```python
from build123d import *

# Parameters (mm, degrees)
SKETCH1_W           = 38.1
SKETCH1_H           = 20.32
BOSS_EXTRUDE1_DEPTH = 8.89
CUT_EXTRUDE3_START  = -20.32
CUT_EXTRUDE3_DEPTH  = 20.32
CUT_EXTRUDE5_DEPTH  = 42.856889745
SKETCH15_R          = 6.9596
CUT_EXTRUDE7_DEPTH  = 31.005753887
CUT_EXTRUDE8_DEPTH  = 3.81


# Read off the part's stored shape, not the designer's step: Cut-Extrude3
with BuildPart() as part:
    # Sketch1 → Boss-Extrude1 (new body)
    with BuildSketch(Plane.XY):
        Rectangle(SKETCH1_W, SKETCH1_H)
    extrude(amount=BOSS_EXTRUDE1_DEPTH)

    # Cut-Extrude3 outline → Cut-Extrude3 (cut)
    with BuildSketch(Plane(origin=(0, 10.16, 0), x_dir=(1, 0, 0), z_dir=(0, 1, 0)).offset(CUT_EXTRUDE3_START)):
        with BuildLine():
            ThreePointArc((19.05, -6.110642457), (9.62584189, -8.191501824), (0, -8.89))
            Line((0, -8.89), (19.05, -8.89))
            Line((19.05, -8.89), (19.05, -6.110642457))
        make_face()
        with BuildLine():
            ThreePointArc((0, -8.89), (-9.62584189, -8.191501824), (-19.05, -6.110642457))
            Line((-19.05, -6.110642457), (-19.05, -8.89))
            Line((-19.05, -8.89), (0, -8.89))
        make_face()
    extrude(amount=CUT_EXTRUDE3_DEPTH, mode=Mode.SUBTRACT)

    # Sketch12 → #6 Clearance Hole2 (revolve, cut)
    with BuildSketch(Plane(origin=(13.00764722, 0, 7.608858571), x_dir=(0.9807852804032313, 0, -0.19509032201612442), z_dir=(0, 1, 0))):
        Polygon((0, 0), (0, 13.840824014), (1.89865, 12.7), (1.89865, 0), align=None)
    f_6_clearance_hole2 = revolve(axis=Axis((14.246470765, 0, 13.836845101), (-0.19509032201612442, 0, -0.9807852804032313)), mode=Mode.SUBTRACT)

    # Sketch14 → Cut-Extrude5 (cut, through all)
    with BuildSketch(Plane(origin=(12.313906035, -17.145, 4.121186114), x_dir=(-0.9807852804032313, 0, 0.19509032201612445), z_dir=(-0.19509032201612445, 0, -0.9807852804032313))):
        Polygon((0, 21.764379504), (-4.0005, 19.454689752), (-4.0005, 14.835310248), (0, 12.525620496), (4.0005, 14.835310248), (4.0005, 19.454689752), align=None)
    cut_extrude5 = extrude(amount=CUT_EXTRUDE5_DEPTH, mode=Mode.SUBTRACT)

    # Mirror1: #6 Clearance Hole2, Cut-Extrude5 across plane
    add(f_6_clearance_hole2.mirror(Plane(origin=(0, 0, 0), x_dir=(0, 0, 1), z_dir=(1, 0, 0))), mode=Mode.SUBTRACT)
    add(cut_extrude5.mirror(Plane(origin=(0, 0, 0), x_dir=(0, 0, 1), z_dir=(1, 0, 0))), mode=Mode.SUBTRACT)

    # Sketch15 → Cut-Extrude7 (cut, through all)
    with BuildSketch(Plane(origin=(-1.163639199, -10.16, 8.879845075), x_dir=(-0.9998476951563913, 0, -0.017452406437284837), z_dir=(0.017452406437284837, 0, -0.9998476951563913))):
        with Locations(Location((0, 10.16, 0), (0, 0, 180))):
            Circle(SKETCH15_R)
    extrude(amount=CUT_EXTRUDE7_DEPTH, mode=Mode.SUBTRACT)

    # Sketch16 → Cut-Extrude8 (cut)
    with BuildSketch(Plane(origin=(-1.163639199, -10.16, 8.879845075), x_dir=(-0.9998476951563913, 0, -0.017452406437284837), z_dir=(0.017452406437284837, 0, -0.9998476951563913))):
        Polygon((-4.934670486, 18.7071), (-9.869340972, 10.16), (-4.934670486, 1.6129), (4.934670486, 1.6129), (9.869340972, 10.16), (4.934670486, 18.7071), align=None)
    extrude(amount=CUT_EXTRUDE8_DEPTH, mode=Mode.SUBTRACT)


solid = part.part
```
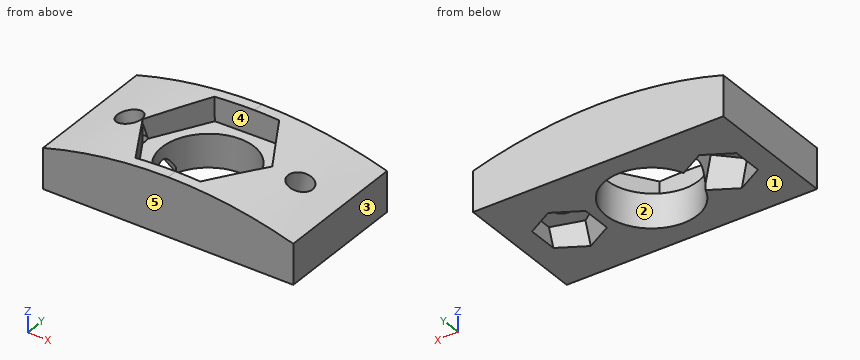
Build history of the part. All positions in model axes, mm. Face numbers are marked on the shaded views. A direction names the side the tool comes from. Round coordinates to 2 decimals unless told otherwise and drop trailing zeros. Order: outer loops, then holes, each group sorted by start corner. A loop starts at its lowest first (then second) coordinate and runs counter-clockwise, first axis right, second up. Notation, with made-up numbers: (20, 58.25) - (77, 58.25) arc R20 cw to (77, 73.25) - close; hole circle Ø1 at (14, 46.5). An arc over 180 degrees is marked (long way). Use a Markdown table: item, result.
1) Flat gauge pins, fed straight in: pin 1 Ø1.5 at (x, y) = (14.5, -2) entering from +Z; pin 2 Ø12 at (x, y) = (-14.5, 6.5) entering from -Z; pin 3 Ø5 at (x, y) = (-4.5, 2) entering from +Z. Where does each tip first touch, or does it go through?
Recorded:
| item | result |
|---|---|
| pin 1 | stops at z = 7.46 |
| pin 2 | stops at z = 0 |
| pin 3 | passes through |
2) Pull direction Y, two halves, no side cores. Call the marked faces 3, 4 and 5: pulls with the +Y half, pulls with the -Y half, needs draft (parallel to the pull), parting line crosses it, or undercut.
Recorded:
| item | result |
|---|---|
| face 3 | needs draft |
| face 4 | undercut |
| face 5 | pulls with the -Y half |
3) Wall check: L1, parallel to X at y = 4.5, z = 2; L2, parallel to X at y = -2.5, z = 2.25; L3, parallel to Y at x = 0.5, z = 8.5. Give the ranges that are in metal, low to high.
Recorded:
| item | result |
|---|---|
| L1 | x = -19.05 to -12.1, -11.68 to -6.35, 4.27 to 11.68, 12.1 to 19.05 |
| L2 | x = -19.05 to -15.68, -8.2 to -7.54, 5.45 to 8.2, 15.68 to 19.05 |
| L3 | y = -10.16 to -8.55, 8.55 to 10.16 |
4) Saw through at C-C on x = 8. Write the cut outline in (y, z), and give its area (3 significant figures).
Recorded:
| item | result |
|---|---|
| outline | (-10.16, 0) - (-2.64, 0) - (-2.31, 2.94) - (2.31, 2.94) - (2.64, 0) - (10.16, 0) - (10.16, 8.41) - (1.24, 8.41) - (1.34, 5.23) - (-1.34, 5.23) - (-1.24, 8.41) - (-10.16, 8.41) - close |
| area | 148 mm² |
5) Tool access for the marked faces 1 and 2: list every direction of +Z, -Z, +X, -X, +Y, -Y with a clear straight run to the whole face (end or side of a thin tool).
Recorded:
| item | result |
|---|---|
| face 1 | -Z, +X, -X, +Y, -Y |
| face 2 | none |
6) Saw through at A-A on y = 1.25. Write the cut outline in (x, z) (3 decimals), and give its area (3 significant figures).
Recorded:
| item | result |
|---|---|
| outline | (-19.05, 0) - (-15.573, 0) - (-16.238, 3.341) - (-13.716, 3.842) - (-14.406, 7.315) arc R66.675 ccw to (-19.05, 6.111) - close; (-11.603, 7.873) - (-10.912, 4.4) - (-8.39, 4.902) - (-7.899, 2.429) - (-7.943, 4.951) - (-10.243, 4.911) - (-10.299, 8.09) arc R66.675 ccw to start; (5.748, 5.19) - (5.839, 0) - (7.415, 0) - (8.39, 4.902) - (10.912, 4.4) - (11.603, 7.873) arc R66.675 ccw to (7.994, 8.409) - (8.049, 5.23) - close; (13.716, 3.842) - (16.238, 3.341) - (15.573, 0) - (19.05, 0) - (19.05, 6.111) arc R66.675 ccw to (14.406, 7.315) - close |
| area | 81.4 mm² |
7) Saw through at D-D on z = 2. Give the number of separate pieces and of enclosed holes in the cut face, and give its area (3 significant figures).
Recorded:
| item | result |
|---|---|
| separate pieces | 1 |
| enclosed holes | 2 |
| area | 509 mm² |
8) Saw through at B-B on y = -3.25. Write the cut outline in (x, z) (3 decimals).
Recorded:
| item | result |
|---|---|
| outline | (-19.05, 0) - (-13.912, 0) - (-14.64, 3.658) - (-9.988, 4.584) - (-9.076, 0) - (-7.164, 0) - (-7.25, 4.963) - (-9.089, 4.931) - (-9.147, 8.26) arc R66.675 ccw to (-19.05, 6.111) - close; (5.056, 5.178) - (5.146, 0) - (9.076, 0) - (9.988, 4.584) - (14.64, 3.658) - (13.912, 0) - (19.05, 0) - (19.05, 6.111) arc R66.675 ccw to (6.836, 8.539) - (6.895, 5.21) - close |
